Source: CAD feature listing. Evaluate the final solid. Frame: model axes, mm. Face numbers are marked on the shaded views. A direction names the side the tool comes from. Give positions to 0.01 mm unless a question says otherwise; leave off trailing zeros. Loops run counter-clockwise (first coordinate to the right, second up) from the corner with the lowest first, then second, coordinate; pieces in that order, holes last. Notation, with made-up numbers: M -33.75,52.25 L -8.75,52.25 A16 cw -8.75,60.25 Z; hole C 87,34.25 d2. An arc over 180 degrees is marked long. Write item = value, one per line.
from build123d import *

# Parameters (mm, degrees)
P_IDAT_VYSUNUT_M2_DEPTH  = 0.8
P_IDAT_VYSUNUT_M3_DEPTH  = 1.5
ZAOBLIT1_R               = 8
ODEBRAT_VYSUNUT_M3_DEPTH = 51.416211215


with BuildPart() as part:
    # Skica1 → Přidat vysunutím2 (new body)
    with BuildSketch(Plane.XY):
        Polygon((24.5, -0.229513463), (-24.5, -0.229513463), (-24.5, 7.770486537), (-23, 7.770486537), (-21.499999864, 11.770486537), (-9.499999864, 11.770486537), (-8, 7.770487265), (8, 7.770487265), (9.499999864, 11.770486537), (21.499999864, 11.770486537), (23, 7.770486537), (24.5, 7.770486537), align=None)
    extrude(amount=P_IDAT_VYSUNUT_M2_DEPTH)

    # Skica2 → Přidat vysunutím3 (add)
    with BuildSketch(Plane(origin=(0, 0, 0), x_dir=(-1, 0, 0), z_dir=(0, 0, -1))):
        Polygon((-23, 7.770486537), (-21.499999864, 11.770486537), (-9.499999864, 11.770486537), (-8, 7.770487265), align=None)
        Polygon((8, 7.770487265), (23, 7.770486537), (21.499999864, 11.770486537), (9.499999864, 11.770486537), align=None)
    extrude(amount=P_IDAT_VYSUNUT_M3_DEPTH)

    # Zaoblit1
    # the kernel refuses this fillet: 8 mm, written as the material it takes off along each edge
    with BuildSketch(Plane(origin=(-4.533442337, 11.770486537, 0.8), x_dir=(0, -1, 0), z_dir=(1, 0, 0)), Plane(origin=(-35.533442064, 11.770486537, 0.8), x_dir=(0, -1, 0), z_dir=(1, 0, 0))) as zaoblit1_piece_1:
        with BuildLine():
            CenterArc((5.61337688, 8), ZAOBLIT1_R, 225.438687956, 44.561312044)
            Line((0, 2.3), (0, 0))
            Line((0, 0), (5.61337688, 0))
        make_face()
    extrude(amount=40.066884401, mode=Mode.SUBTRACT)

    # Skica7 → Odebrat vysunutím3 (cut, through all)
    with BuildSketch(Plane(origin=(24.5, 0, 0), x_dir=(0, 0, -1), z_dir=(1, 0, 0))):
        with BuildLine():
            Line((0, 7.739922094), (1.948215566, 7.739922094))
            Line((1.948215566, 7.739922094), (1.948215566, 12.51596757))
            add(Edge.make_bspline(
                [(0, 7.739922094), (0.473258475, 10.37513305), (1.948215566, 12.51596757)],
                knots=[0, 0, 0, 1, 1, 1], degree=2))
        make_face()
    extrude(amount=-ODEBRAT_VYSUNUT_M3_DEPTH, mode=Mode.SUBTRACT)


solid = part.part
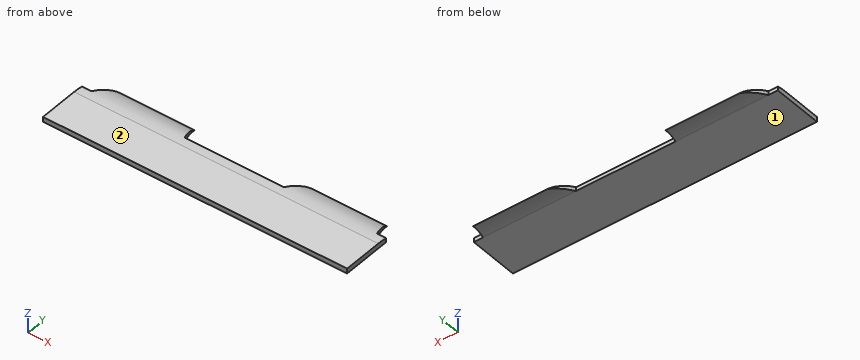
1. First-contact query: pin 1 Ø0.5 at (x, z) = (24, 0.5) entering from +Y; pin 2 Ø1.5 at (x, y) = (-4.5, 7) entering from -Z. Flat tips, straight axial feed; report the tip coordinate or a pass-through.
Derived:
pin_1 = 7.77
pin_2 = 0
2. Cut plane A-A, the plane x = 3. Return the cut outline in (y, z).
Derived:
outline = M -0.23,0 L 7.77,0 L 7.77,0.64 A8 ccw 6.16,0.8 L -0.23,0.8 Z
3. Cut plane B-B, the plane y = 5.25. Return the cut outline in (x, z), then the cut area to 3 significant figures.
Derived:
outline = M -24.5,0 L 24.5,0 L 24.5,0.8 L -24.5,0.8 Z
area = 39.2 mm²
4. Reachability of the marked faces 1 and 2 from +Z, -Z, +X, -X, +Y, -Y: full face, straight path, thin tool, end or side. Return the list, or none.
Derived:
face_1 = -Z, +X, -X, -Y
face_2 = +Z, +X, -X, +Y, -Y
5. Material intervals for probe 1 along Z at (x, y) = (-7.5, 1.5); probe 2 along Y at (x, z) = (6, 0.1); probe 3 along Z at (x, y) = (18, 7.75), sorted ascending. Write a range as from..to.
Derived:
probe_1 = 0..0.8
probe_2 = -0.23..7.77
probe_3 = 0..0.64
